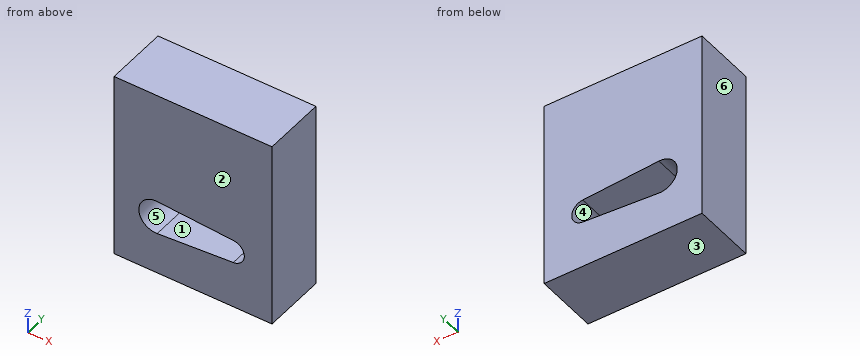
from build123d import *

# Parameters (mm, degrees)
F0_W          = 127
F0_H          = 152.4
F1_DEPTH      = 25.4
F1_DEPTH_BACK = 25.4
F3_DEPTH      = 50.801


with BuildPart() as f1:
    # F0 (on Front) → F1 (new body, two sides)
    with BuildSketch(Plane.XZ) as f1_sk:
        with Locations((63.5, 76.2)):
            Rectangle(F0_W, F0_H)
    extrude(amount=F1_DEPTH)
    extrude(f1_sk.sketch, amount=-F1_DEPTH_BACK)

    # F2 (on face) → F3 (cut, through all)
    with BuildSketch(Plane.XZ.offset(25.4)):
        with BuildLine():
            Line((34.656941, 33.802745), (95.884816, 38.070348))
            ThreePointArc((95.884816, 38.070348), (104.736954, 47.56096), (95.884816, 57.051572))
            Line((95.884816, 57.051572), (34.656941, 61.319176))
            ThreePointArc((34.656941, 61.319176), (19.906394, 47.56096), (34.656941, 33.802745))
        make_face()
    extrude(amount=-F3_DEPTH, mode=Mode.SUBTRACT)


solid = f1.part
Read the model definition and answer for the solid it produces. Units are mm, in the model's axes. Face numbers are marked on the shaded views. A direction names the side the tool comes from. Round coordinates to 2 decimals unless told otherwise and drop trailing zeros. Write each loop counter-clockwise with the first axis right and the second up, starting at its lowest first coordinate (ties: lowest second). Pieces come first, ordered by that corner, then holes. Notation, with made-up numbers: (69.5, 57.25) - (89.5, 57.25) arc R24 cw to (89.5, 78.25) - close; hole circle Ø9 at (53, 9). An arc over 180 degrees is marked (long way). Use a Markdown table: item, result.
(1) Straight lines are drawn through the part: line 1 along Z through (x, y) = (58.5, -22); line 2 along X through (y, z) = (-14, 41); line 3 along Z through (x, y) = (85, 5.5). For each, find the intervals that lie inside material, in ascending order. Write a range as [from, to].
Reported:
| item | result |
|---|---|
| line 1 | [0, 35.46], [59.66, 152.4] |
| line 2 | [0, 21.57], [102.11, 127] |
| line 3 | [0, 37.31], [57.81, 152.4] |
(2) The part is cut by section C-C (x = 87). Write down the section's boundary in (y, z), then the cut area to 3 significant figures.
Reported:
| item | result |
|---|---|
| outline | (-25.4, 0) - (25.4, 0) - (25.4, 37.45) - (-25.4, 37.45) - close; (-25.4, 57.67) - (25.4, 57.67) - (25.4, 152.4) - (-25.4, 152.4) - close |
| area | 6,710 mm2 |
(3) The mould has two halves that part along Z. Classify the marked faces 1, 2, 3 and 4: released by +Z, released by -Z, zero draft, split by the parting line, or undercut.
Reported:
| item | result |
|---|---|
| face 1 | undercut |
| face 2 | zero draft |
| face 3 | released by -Z |
| face 4 | undercut |
(4) The part is cut by section B-B (x = 62.5). Write down the section's boundary in (y, z), then the cut area to 3 significant figures.
Reported:
| item | result |
|---|---|
| outline | (-25.4, 0) - (25.4, 0) - (25.4, 35.74) - (-25.4, 35.74) - close; (-25.4, 59.38) - (25.4, 59.38) - (25.4, 152.4) - (-25.4, 152.4) - close |
| area | 6,540 mm2 |
(5) The part is cut by section A-A (y = 15.5). Write down the section's boundary in (x, z), then the cut area to 3 significant figures.
Reported:
| item | result |
|---|---|
| outline | (0, 0) - (127, 0) - (127, 152.4) - (0, 152.4) - close; hole (34.66, 33.8) - (95.88, 38.07) arc R9.51 ccw to (95.88, 57.05) - (34.66, 61.32) arc R13.79 ccw (long way) to start |
| area | 17,500 mm2 |
(6) Which of the six approach directions +Z, -Z, +X, -X, +Y, -Y give full straight-line access (tool end or side, diameter ignored) to the marked faces 5 and 6?
Reported:
| item | result |
|---|---|
| face 5 | +Y, -Y |
| face 6 | +Z, -Z, -X, +Y, -Y |
